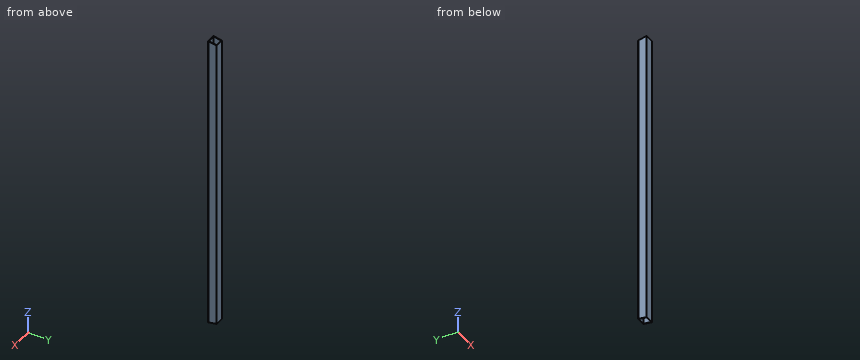
```python
from build123d import *

# Parameters (mm, degrees)
SKETCH_W     = 25
SKETCH_H     = 25
SKETCH_W_2   = 22
SKETCH_H_2   = 22
PAD_DEPTH    = 882
FILLET_R     = 0.74
POCKET_DEPTH = 25.001


with BuildPart() as part:
    # Sketch → Pad (new body)
    with BuildSketch(Plane.XY):
        with Locations((12.5, 12.5)):
            Rectangle(SKETCH_W, SKETCH_H)
        with Locations((12.5, 12.5)):
            Rectangle(SKETCH_W_2, SKETCH_H_2, mode=Mode.SUBTRACT)
    extrude(amount=PAD_DEPTH)

    # Fillet
    fillet_edges = [part.edges().sort_by_distance(p)[0] for p in [
        (25, 0, 441),
        (0, 0, 441),
        (25, 25, 441),
        (0, 25, 441),
    ]]
    fillet(fillet_edges, radius=FILLET_R)

    # Sketch001 (on Face6 of Fillet) → Pocket (cut, through all)
    with BuildSketch(Plane(origin=(0, 0, 0), x_dir=(0, -1, 0), z_dir=(-1, 0, 0))):
        Polygon((0, 882), (-46.854502, 873.738287), (-48.019741, 909.975952), align=None)
        Polygon((0, 0), (-35.255848, -14.284037), (-39.064261, 6.888083), align=None)
    extrude(amount=-POCKET_DEPTH, mode=Mode.SUBTRACT)


solid = part.part
```
CAD build for the part. Positions are in the model's coordinates, mm. Coordinates: 2 decimals unless noted, no trailing zeros. Order: outer loops, then holes, each group sorted by start corner. A loop starts at its lowest first (then second) coordinate and runs counter-clockwise, first axis right, second up. Notation, with made-up numbers: M 46.5,29 L 68.5,29 A16 ccw 68.5,53 Z; hole C 56,45 d5. An arc over 180 degrees is marked long. Answer as CSV lines item,"result".
1) Flat gauge pin, fed straight in: P1, Ø12, axis at x = 21.5, y = 5.5, coming from the +Z side. Where does the tip first touch, or does it go through?
Verdict:
P1,"z = 882"
2) Cut at C-C (y = 5.75). List the corners of the cut face in (x, z), then the cut area to 3 significant figures.
Verdict:
outline,"M 0,1.01 L 1.5,1.01 L 1.5,880.99 L 0,880.99 Z; M 23.5,1.01 L 25,1.01 L 25,880.99 L 23.5,880.99 Z"
area,"2,640 mm2"
3) Drill centre line: L1, parallel to Y at x = 14.5, z = 836.5. Where is it in solid material? Low to high. Write a range as from..to.
Verdict:
L1,"0..1.5, 23.5..25"
4) Cut at B-B (x = 12). List the corners of the cut face in (y, z), then the cut area to 3 significant figures.
Verdict:
outline,"M 0,0 L 1.5,0.26 L 1.5,881.74 L 0,882 Z; M 23.5,4.14 L 25,4.41 L 25,877.59 L 23.5,877.86 Z"
area,"2,630 mm2"
5) Cut at A-A (z = 517). List the corners of the cut face in (x, y), then the cut area to 3 significant figures.
Verdict:
outline,"M 0,0.74 A0.74 ccw 0.74,0 L 24.26,0 A0.74 ccw 25,0.74 L 25,24.26 A0.74 ccw 24.26,25 L 0.74,25 A0.74 ccw 0,24.26 Z; hole M 1.5,1.5 L 23.5,1.5 L 23.5,23.5 L 1.5,23.5 Z"
area,"141 mm2"
